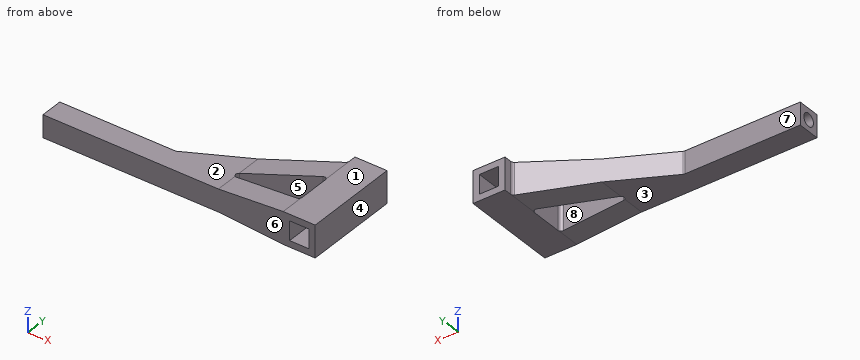
Autodesk Inventor part; units mm, degrees
ref_plane "YZ Plane" through (0, 0, 0) normal (1, 0, 0) x (0, 1, 0)
ref_plane "XZ Plane" through (0, 0, 0) normal (0, 1, 0) x (-1, 0, 0)
ref_plane "XY Plane" through (0, 0, 0) normal (0, 0, 1) x (1, 0, 0)
sketch "Sketch1" plane through (0, 0, 0) normal (0, 1, 0) x (-1, 0, 0)
  line L0 (0, 0) -> (10, 0)
  line L1 (10, 0) -> (10, -10)
  line L2 (10, -10) -> (0, -10)
  line L3 (0, -10) -> (0, 0)
  line L4 (10, 0) -> (0, -10) construction
  line L5 (10, -10) -> (0, 0) construction
  line L6 (2, -2) -> (8, -2)
  line L7 (8, -2) -> (8, -8)
  line L8 (8, -8) -> (2, -8)
  line L9 (2, -8) -> (2, -2)
  line L10 (2, -2) -> (8, -8) construction
  line L11 (8, -2) -> (2, -8) construction
  point P0 (5, -5)
  dimension "d0" = 10
  dimension "d4" = 6
  dimension "d5" = 6
extrude "Extrusion1" add sketch "Sketch1" along normal blind 30
sketch "Sketch2" plane through (-10, 0, -10) normal (-1, 0, 0) x (0, 0, 1)
  line L0 (0, 30) -> (10, 30) construction
  line L1 (10, 0) -> (0, 0)
  line L2 (10, 0) -> (0, 0) construction
  line L3 (0, 0) -> (0, 7)
  line L4 (0, 7) -> (10, 7)
  line L5 (10, 7) -> (10, 0)
  line L6 (0, 0) -> (0, 30) construction
  line L7 (10, 0) -> (10, 30) construction
  dimension "d8" = 7
  dimension "d9" = 10
extrude "Extrusion2" add sketch "Sketch2" along normal blind 75
chamfer "Chamfer1" distance 20 distance2 38.75 1 edges at (-10, 7, -5) measured on face at (-10, 14.6667, -6.6667)
sketch "Sketch3" plane through (0, 0, 0) normal (0, 0, 1) x (1, 0, 0)
  line L0 (-48.75, 7) -> (-85, 7) construction
  line L1 (-10, 27) -> (-10, 30) construction
  line L2 (-9.9219, 6.8486) -> (-33.7809, 6.8486)
  line L3 (-33.7809, 6.8486) -> (-9.9219, 19.163)
  line L4 (-9.9219, 19.163) -> (-9.9219, 6.8486)
  line L5 (-48.75, 7) -> (-10, 27)
  point P0 (0, 0)
  dimension "d21" = 7
extrude "Extrusion3" cut sketch "Sketch3" against normal through all
sketch "Sketch6" plane through (0, 0, 0) normal (0, -1, 0) x (1, 0, 0)
  line L0 (-85, -10) -> (-85, 0) construction
  line L1 (-85, -5) -> (0, -5) construction
  line L2 (0, 0) -> (0, -10) construction
  line L3 (-30.2304, -1.5) -> (-85, -1.5)
  line L4 (-85, -1.5) -> (-85, -8.5)
  line L5 (-85, -8.5) -> (-30.2304, -8.5)
  line L6 (-30.2304, -8.5) -> (-30.2304, -1.5) construction
  line L7 (-30.2304, -1.5) -> (-85, -8.5) construction
  line L8 (-85, -1.5) -> (-30.2304, -8.5) construction
  line L9 (-30.2304, -8.5) -> (0, -8.5) construction
  line L10 (-30.2304, -1.5) -> (0, -1.5) construction
  line L11 (-30.2304, -8.5) -> (-10, -10)
  line L12 (0, -10) -> (-10, -10) construction
  line L13 (-30.2304, -1.5) -> (-10, 0)
  line L14 (-10, 0) -> (0, 0) construction
  line L15 (-10, -10) -> (-10, -18.6026)
  line L16 (-10, -18.6026) -> (-95.3433, -18.6026)
  line L17 (-95.3433, -18.6026) -> (-95.3433, 10.4)
  line L18 (-95.3433, 10.4) -> (-10, 10.4)
  line L19 (-10, 10.4) -> (-10, 0)
  point P0 (-57.6152, -5)
  dimension "d22" = 7
extrude "Extrusion5" cut sketch "Sketch6" against normal through all
hole "Hole1" at (-85, 3.5, -5) direction (1, 0, 0) diameter 4 depth 5
fillet "Fillet1" radius 1 5 edges at (-33.7809, 6.8486, -5) (-9.9219, 6.8486, -5) (-9.9219, 19.163, -5) (-48.75, 7, -5) (-10, 27, -5)
properties part number "foot_1_2"
Work out the finished part from the listing and answer in its coordinate system (mm). Face numbers are marked on the shaded views. A direction names the side the tool comes from. Give positions to 0.01 mm unless a question says otherwise; leave off trailing zeros. Loops run counter-clockwise (first coordinate to the right, second up) from the corner with the lowest first, then second, coordinate; pieces in that order, holes last. Notation, with made-up numbers: (-34, 32) -> (9, 32) arc R27 cw to (9, 59) -> close; hole circle Ø5 at (-37, 56.25). An arc over 180 degrees is marked (long way). Put each result on its own line as item: value. Start each with the question number.
Item 1: Find the intervals of material crossed by L1, parallel to Y at x = -81, z = -5; L2, parallel to Z at x = -82.6, y = 3.5; L3, parallel to X at y = 8.5, z = -2.75, in increasing order. Write a range as [from, to].
Item 2: Each of these flat-tipped pins is pushed along its axis until it touches: P1, Ø0.7, axis at y = 28.5, z = -3.5, coming from the -X side; P2, Ø4, axis at x = -49, z = -2, coming from the +Y side; P3, Ø18, axis at x = -60.5, y = 10.5, coming from the +Z side. Where does it stop, or does it pass through?
Item 3: Which of the six approach directions +Z, -Z, +X, -X, +Y, -Y give full straight-line access (tool end or side, diameter ignored) to the marked faces 1, 2, 3, 4 and 5?
Item 4: The part is cut by section A-A (z = -5). Give the vertices of the cut face in (x, y), then the cut area to 3 significant figures.
Item 5: The part is cut by section C-C (x = -23). Give the vertices of the cut face in (y, z).
Item 6: The part is cut by section B-B (y = 3.5). Give the vertices of the cut face in (x, z), then the cut area to 3 significant figures.
Item 7: The part is cut by section D-D (y = 9.75). Give the vertices of the cut face in (x, z), then the cut area to 3 significant figures.
Item 8: The mould has two halves that part along Y. Classify the marked faces 6, 7 and 8: released by +Y, released by -Y, zero draft, split by the parting line, or undercut.
Answers below:
1. L1: [0, 1.5], [5.5, 7]
1. L2: [-8.5, -7], [-3, -1.5]
1. L3: [-45.84, -30.42], [-9.92, -8], [-2, 0]
2. P1: x = -10
2. P2: y = 7.9
2. P3: z = -1.5
3. face 1: +Z, +X, -X, +Y, -Y
3. face 2: +Z, -X, +Y, -Y
3. face 3: -Z, -X, +Y, -Y
3. face 4: +Z, -Z, +X, +Y, -Y
3. face 5: +Z, -Z
4. outline: (-85, 0) -> (-8, 0) -> (-8, 30) -> (-10, 30) -> (-10, 27.61) arc R1 cw to (-10.54, 26.72) -> (-48.53, 7.11) arc R1 cw to (-48.99, 7) -> (-85, 7) -> (-85, 5.5) -> (-80, 5.5) -> (-80, 1.5) -> (-85, 1.5) -> close; (-2, 0) -> (0, 0) -> (0, 30) -> (-2, 30) -> close; hole (-30.12, 8.74) arc R1 ccw to (-29.66, 6.85) -> (-10.92, 6.85) arc R1 ccw to (-9.92, 7.85) -> (-9.92, 17.52) arc R1 ccw to (-11.38, 18.41) -> close
4. area: 869 mm2
5. outline: (0, -9.04) -> (6.85, -9.04) -> (6.85, -0.96) -> (0, -0.96) -> close; (12.41, -9.04) -> (20.29, -9.04) -> (20.29, -0.96) -> (12.41, -0.96) -> close
6. outline: (-85, -8.5) -> (-30.23, -8.5) -> (-10, -10) -> (0, -10) -> (0, 0) -> (-10, 0) -> (-30.23, -1.5) -> (-85, -1.5) -> (-85, -3) -> (-80, -3) -> (-80, -7) -> (-85, -7) -> close; hole (-8, -8) -> (-2, -8) -> (-2, -2) -> (-8, -2) -> close
6. area: 599 mm2
7. outline: (-43.42, -8.5) -> (-30.23, -8.5) -> (-28.16, -8.65) -> (-28.16, -1.35) -> (-30.23, -1.5) -> (-43.42, -1.5) -> close; (-9.92, -10) -> (0, -10) -> (0, 0) -> (-9.92, 0) -> close; hole (-8, -8) -> (-2, -8) -> (-2, -2) -> (-8, -2) -> close
7. area: 170 mm2
8. face 6: released by -Y
8. face 7: released by +Y
8. face 8: undercut
